The model under review builds one solid part; all positions refer to its coordinate system, in mm. A direction names the side the tool comes from. Coordinates: 2 decimals unless noted, no trailing zeros. Loops run counter-clockwise (first coordinate to the right, second up) from the corner with the lowest first, then second, coordinate; pieces in that order, holes last. Notation, with made-up numbers: M 55.25,-26.75 L 60.25,-26.75 A7 ccw 60.25,-13.75 Z; hole C 88.25,22.25 d2. An arc over 180 degrees is marked long. Write item = value, one per line. Start each with the question number.
Q1. We need section C-C on x = 19. Give the boundary of the cut face in (y, z), and give its area (4 significant figures).
Q2. Clearance check with flat-ended pins moving along their axes: pin 1 Ø6 at (x, z) = (144, 17) entering from -Y; pin 2 Ø2 at (y, z) = (26.5, 11.5) entering from +X; pin 3 Ø4 at (x, y) = (4, 4) entering from +Z; pin 4 Ø1.8 at (x, y) = (206, 4) entering from +Z. State where each tip first meets the part, or that it passes through.
Q3. Mouldability with a two-part tool opening along Y and no side actions: class faces 4 (the face through (104, 87.5, 12)), 5 (the face through (97, 5, 2.5)), 6 (the face through (104, 85, 13)) as released by +Y, released by -Y, zero draft, split by the parting line, or undercut.
Q4. We need section B-B on y = 62. Give the boundary of the cut face in (x, z), and give its area (3 significant figures).
Q5. We need section A-A on z = 6. Give the boundary of the cut face in (x, y).
Q6. Wall thickness on probe 1 along Y at (x, z) = (142.5, 11.75); probe 2 along Y at (x, z) = (4, 0.85); probe 3 along X at (y, z) = (91, 1.95): over which ranges is each line inside the solid? List them lowest first.
Q7. For faces 1 (the face through (7.5, 47, 12)), 2 (the face through (104, 7.5, 12)), 3 (the face through (10, 47, 13)), list the 3-axis set-ups (+Z, -Z, +X, -X, +Y, -Y) from which the entire face can be reached by the end or side of a thin tool; tool diameter is ignored.
from build123d import *

# Parameters (mm, degrees)
SKETCH1_W           = 210
SKETCH1_H           = 95
BOSS_EXTRUDE1_DEPTH = 2.5
SKETCH2_W           = 195
SKETCH2_H           = 80
BOSS_EXTRUDE2_DEPTH = 20
SKETCH3_W           = 190
SKETCH3_H           = 75
CUT_EXTRUDE1_DEPTH  = 20
SKETCH5_W           = 15
SKETCH5_H           = 5
CUT_EXTRUDE3_DEPTH  = 80
SKETCH6_R           = 1.5
CUT_EXTRUDE4_DEPTH  = 2.5


with BuildPart() as part:
    # Sketch1 → Boss-Extrude1 (new body)
    with BuildSketch(Plane.XY):
        with Locations((105, 47.5)):
            Rectangle(SKETCH1_W, SKETCH1_H)
    extrude(amount=BOSS_EXTRUDE1_DEPTH)

    # Sketch2 → Boss-Extrude2 (add)
    with BuildSketch(Plane.XY.offset(2.5)):
        with Locations((105, 47.5)):
            Rectangle(SKETCH2_W, SKETCH2_H)
    extrude(amount=BOSS_EXTRUDE2_DEPTH)

    # Sketch3 → Cut-Extrude1 (cut)
    with BuildSketch(Plane.XY.offset(22.5)):
        with Locations((105, 47.5)):
            Rectangle(SKETCH3_W, SKETCH3_H)
    extrude(amount=-CUT_EXTRUDE1_DEPTH, mode=Mode.SUBTRACT)

    # Sketch5 → Cut-Extrude3 (cut)
    with BuildSketch(Plane(origin=(0, 87.5, 0), x_dir=(1, 0, 0), z_dir=(0, 1, 0))):
        with Locations((175, -15)):
            Rectangle(SKETCH5_W, SKETCH5_H)
        with Locations((35, -15)):
            Rectangle(SKETCH5_W, SKETCH5_H)
    extrude(amount=-CUT_EXTRUDE3_DEPTH, mode=Mode.SUBTRACT)

    # Sketch6 → Cut-Extrude4 (cut)
    with BuildSketch(Plane.XY.offset(2.5)):
        with Locations((4, 91)):
            Circle(SKETCH6_R)
        with Locations((206, 91)):
            Circle(SKETCH6_R)
        with Locations((206, 4)):
            Circle(SKETCH6_R)
        with Locations((4, 4)):
            Circle(SKETCH6_R)
    extrude(amount=-CUT_EXTRUDE4_DEPTH, mode=Mode.SUBTRACT)


solid = part.part
Returned:
q1.outline = M 0,0 L 95,0 L 95,2.5 L 87.5,2.5 L 87.5,22.5 L 85,22.5 L 85,2.5 L 10,2.5 L 10,22.5 L 7.5,22.5 L 7.5,2.5 L 0,2.5 Z
q1.area = 337.5 mm^2
q2.pin_1 = 7.5
q2.pin_2 = 202.5
q2.pin_3 = 2.5
q2.pin_4 = through
q3.face_4 = released by +Y
q3.face_5 = zero draft
q3.face_6 = undercut
q4.outline = M 0,0 L 210,0 L 210,2.5 L 202.5,2.5 L 202.5,22.5 L 200,22.5 L 200,2.5 L 10,2.5 L 10,22.5 L 7.5,22.5 L 7.5,2.5 L 0,2.5 Z
q4.area = 625 mm^2
q5.outline = M 7.5,7.5 L 202.5,7.5 L 202.5,87.5 L 7.5,87.5 Z; hole M 10,10 L 200,10 L 200,85 L 10,85 Z
q6.probe_1 = 7.5 to 10, 85 to 87.5
q6.probe_2 = 0 to 2.5, 5.5 to 89.5, 92.5 to 95
q6.probe_3 = 0 to 2.5, 5.5 to 204.5, 207.5 to 210
q7.face_1 = +Z, -X, +Y, -Y
q7.face_2 = +Z, +X, -X, -Y
q7.face_3 = +Z
